Part print with two shaded views. Sizes in mm from the minimum x, y, z corner. A direction names the side the tool comes from. Give positions to 0.01 mm unless a question says otherwise; leave off trailing zeros. Write each loop counter-clockwise with the first axis right and the second up, starting at its lowest first coordinate (ties: lowest second). Pieces come first, ordered by that corner, then holes. Notation, with made-up numbers: (49.5, 9.25) -> (94.5, 9.25) arc R19 ccw to (94.5, 31.25) -> close; hole circle Ø6 at (11.5, -11). An arc over 180 degrees is marked (long way). Answer in a Markdown table with one row per item. Add a question column.
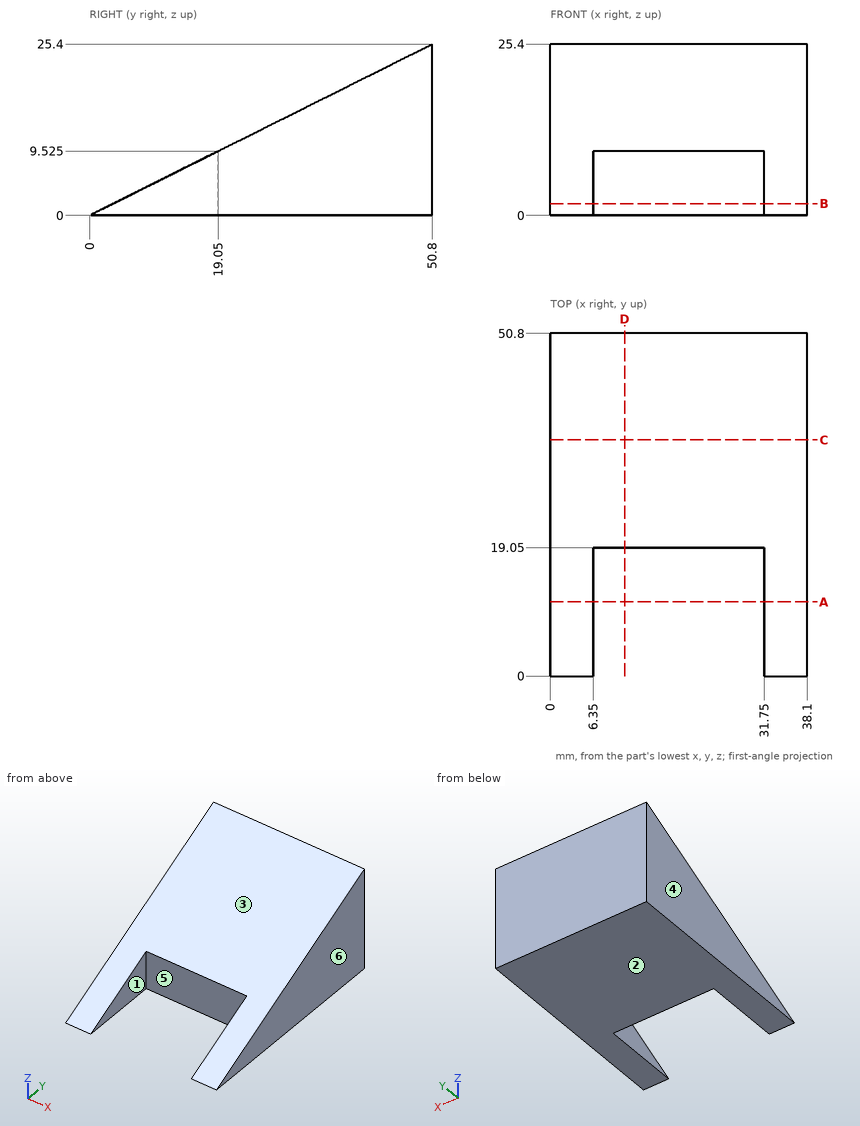
Item 1: Probe L1, parallel to X at y = 14.5, z = 4.25; L2, parallel to Y at x = 36, z = 16.5; L3, parallel to Y at x = 2.5, z = 10. List the from-to ranges inside material, lowest first. Write a range as from..to.
Item 2: Slice it at B-B, the plane z = 1.75. List the corners of the cut face in (x, y).
Item 3: Mould opens along X. For the marked faces 3, 4, 5 and 6 say: released by +X, released by -X, zero draft, split by the parting line, or undercut.
Item 4: Slice it at C-C, the plane y = 35. List the corners of the cut face in (x, z), then the cut area to 3 significant figures.
Item 5: Which spindle directions (+Z, -Z, +X, -X, +Y, -Y) get a long thin tool onto all of the face, cutting with end or side? Do the marked faces 1 and 2. Say none if no direction does.
Item 6: Slice it at A-A, the plane y = 11. List the corners of the cut face in (x, z).
Item 7: Drop flat-ended pins along their axis: pin 1 Ø8 at (x, y) = (28.5, 26) entering from +Z; pin 2 Ø5 at (x, z) = (19.5, 6) entering from -Y. Give the stop position or say it passes through.
Item 8: Slice it at D-D, the plane x = 11. List the corners of the cut face in (y, z) (3 decimals).
Answer key:
| question | item | result |
|---|---|---|
| 1 | L1 | x = 0..6.35, 31.75..38.1 |
| 1 | L2 | y = 33..50.8 |
| 1 | L3 | y = 20..50.8 |
| 2 | outline | (0, 3.5) -> (6.35, 3.5) -> (6.35, 19.05) -> (31.75, 19.05) -> (31.75, 3.5) -> (38.1, 3.5) -> (38.1, 50.8) -> (0, 50.8) -> close |
| 3 | face 3 | zero draft |
| 3 | face 4 | released by -X |
| 3 | face 5 | undercut |
| 3 | face 6 | released by +X |
| 4 | outline | (0, 0) -> (38.1, 0) -> (38.1, 17.5) -> (0, 17.5) -> close |
| 4 | area | 667 mm² |
| 5 | face 1 | +Z, -Z, -Y |
| 5 | face 2 | -Z, +X, -X, +Y, -Y |
| 6 | outline | (0, 0) -> (6.35, 0) -> (6.35, 5.5) -> (0, 5.5) -> close; (31.75, 0) -> (38.1, 0) -> (38.1, 5.5) -> (31.75, 5.5) -> close |
| 7 | pin 1 | stops at z = 15 |
| 7 | pin 2 | stops at y = 19.05 |
| 8 | outline | (19.05, 0) -> (50.8, 0) -> (50.8, 25.4) -> (19.05, 9.525) -> close |
